Part print with two shaded views. Sizes in mm from the minimum x, y, z corner. A direction names the side the tool comes from. Coordinates: 2 decimals unless noted, no trailing zeros. Write each loop counter-clockwise with the first axis right and the second up, starting at its lowest first coordinate (ties: lowest second). Pieces come first, ordered by that corner, then holes. Notation, with made-up numbers: (-30, 71.25) - (-1, 71.25) arc R22 cw to (-1, 91.25) - close; hole circle Ø9 at (12, -28). An arc over 180 degrees is marked (long way). One line per question, with ' | ' between items. Start each with the question number.
1. Flat gauge pins, fed straight in: P1, Ø2, axis at x = 8, z = 22, coming from the +Y side; P2, Ø5, axis at x = 23.5, y = 27.75, coming from the +Z side; P3, Ø1.5, axis at y = 15.5, z = 15, coming from the -X side. Where does each tip first touch, or does it go through?
2. Which spindle directions (+Z, -Z, +X, -X, +Y, -Y) get a long thin tool onto all of the face, cutting with end or side? Do the marked faces 4, 5, 6 and 7. Say none if no direction does.
3. Band-saw the part on D-D, the plane z = 21.5. Write the cut outline in (x, y).
4. Band-saw the part on A-A, the plane y = 4.25. Write the cut outline in (x, z) (3 decimals), then the cut area to 3 significant figures.
5. Two-plate mould, pull along Y, no slides. Class the marked faces 1, 2 and 3: +Y half, -Y half, draft (parallel to the pull), parting line (faces both ways), or undercut.
6. Band-saw the part on B-B, the plane x = 4.5. Write the cut outline in (y, z) (3 decimals).
7. Probe line 1 (Y direction, x = 23.5, z = 2.2) (3 decimals); line 2 (X direction, y = 21.5, z = 32.5); line 3 (Z direction, x = 19.5, y = 29). List the from-to ranges inside material, lowest first.
8. Band-saw the part on C-C, the plane y = 23. Write the cut outline in (x, z), then the cut area to 3 significant figures.
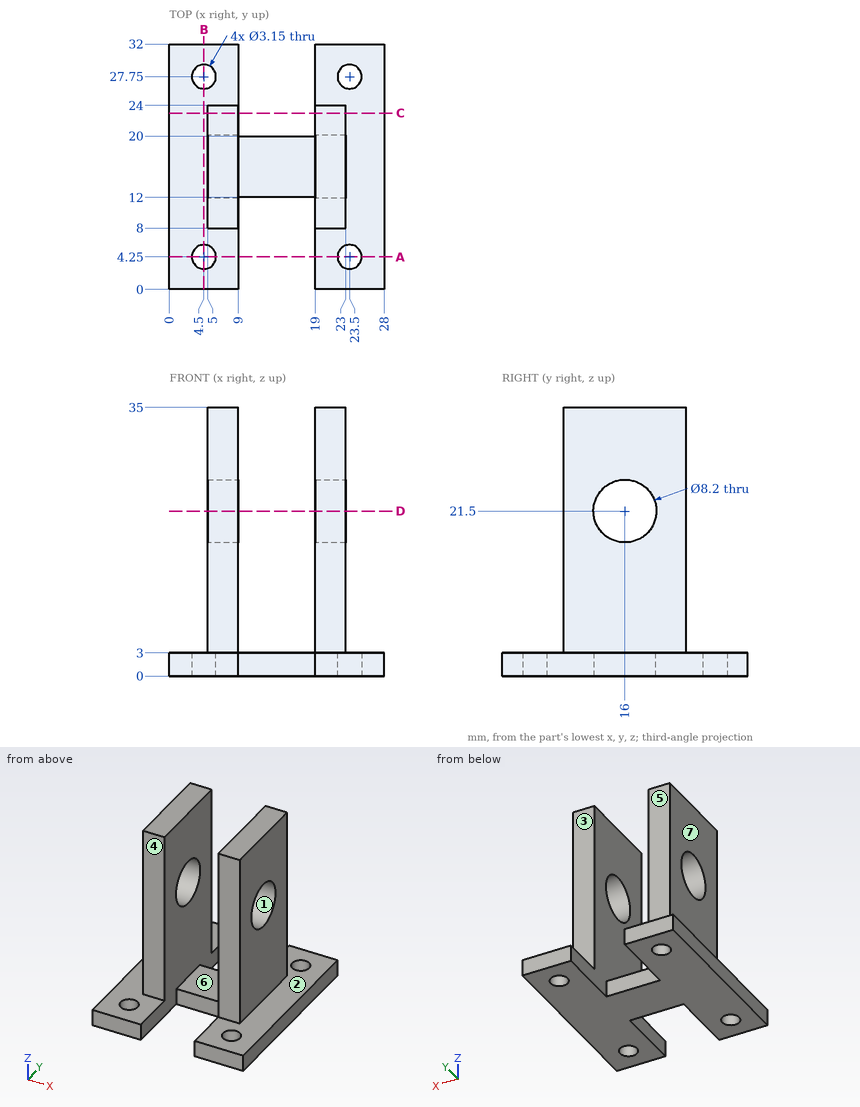
Filled in:
1) P1: stops at y = 24 | P2: stops at z = 3 | P3: stops at x = 5
2) face 4: +Z, +X, -X, -Y | face 5: +Z, +X, -X, +Y | face 6: +Z, +Y, -Y | face 7: +Z, -X, +Y, -Y
3) outline: (5, 8) - (9, 8) - (9, 11.9) - (5, 11.9) - close; (5, 20.1) - (9, 20.1) - (9, 24) - (5, 24) - close; (19, 8) - (23, 8) - (23, 11.9) - (19, 11.9) - close; (19, 20.1) - (23, 20.1) - (23, 24) - (19, 24) - close
4) outline: (0, 0) - (2.925, 0) - (2.925, 3) - (0, 3) - close; (6.075, 0) - (9, 0) - (9, 3) - (6.075, 3) - close; (19, 0) - (21.925, 0) - (21.925, 3) - (19, 3) - close; (25.075, 0) - (28, 0) - (28, 3) - (25.075, 3) - close | area: 35.1 mm²
5) face 1: undercut | face 2: draft | face 3: +Y half
6) outline: (0, 0) - (2.675, 0) - (2.675, 3) - (0, 3) - close; (5.825, 0) - (26.175, 0) - (26.175, 3) - (5.825, 3) - close; (29.325, 0) - (32, 0) - (32, 3) - (29.325, 3) - close
7) line 1: y = 0 to 2.675, 5.825 to 26.175, 29.325 to 32 | line 2: x = 5 to 9, 19 to 23 | line 3: z = 0 to 3
8) outline: (0, 0) - (9, 0) - (9, 35) - (5, 35) - (5, 3) - (0, 3) - close; (19, 0) - (28, 0) - (28, 3) - (23, 3) - (23, 35) - (19, 35) - close | area: 310 mm²
